Model file for the job. Use its own axes, mm. A direction names the side the tool comes from. Give positions to 0.01 mm unless a question says otherwise; leave off trailing zeros. Order: outer loops, then holes, each group sorted by start corner. A loop starts at its lowest first (then second) coordinate and runs counter-clockwise, first axis right, second up. Notation, with made-up numbers: (3.25, -21.5) -> (54.25, -21.5) arc R20 cw to (54.25, 4.5) -> close; hole circle Ø10 at (64.5, -9). An arc over 180 degrees is marked (long way). Answer in a Markdown table with one row per item. Add a question column.
from build123d import *

# Parameters (mm, degrees)
F0_W     = 20
F0_H     = 20
F0_W_2   = 10
F0_H_2   = 10
F1_DEPTH = 2.5
F2_ANGLE = 90


with BuildPart() as f1:
    # F0 (on Front) → F1 (new body)
    with BuildSketch(Plane.XZ):
        Rectangle(F0_W, F0_H)
        Rectangle(F0_W_2, F0_H_2, mode=Mode.SUBTRACT)
    extrude(amount=F1_DEPTH)


with BuildPart() as f1_1:
    # F2: moved
    add(f1.part.rotate(Axis((0, -2.5, 10), (-1, 0, 0)), F2_ANGLE))


solid = f1_1.part
Item 1: Which spindle directions (+Z, -Z, +X, -X, +Y, -Y) get a long thin tool onto all of the face, cutting with end or side? Do faces 5 (the flat face through (0, -17.5, 9)), 6 (the flat face through (0, -6, 7.5)). Say none if no direction does.
Item 2: Saw through at A-A on x = 1. List the corners of the cut face in (y, z).
Item 3: Saw through at B-B on z = 9.4. List the corners of the cut face in (x, y), plus the area to 3 significant figures.
Item 4: Wall check: line 1 (X direction, y = -8.25, z = 9.05); line 2 (Y direction, x = -2, z = 9.05). Give the ranges that are in metal, low to high.
Item 5: Saw through at C-C on y = -10.75. List the corners of the cut face in (x, z).
Item 6: Two-plate mould, pull along Y, no slides. Class faces 1 (the flat face through (0, -2.5, 9)), 2 (the flat face through (-10, -13, 9)), 3 (the flat face through (-5, -13, 9)), 4 (the flat face through (0, -7.5, 9)): pulls with the +Y half, pulls with the -Y half, needs draft (parallel to the pull), parting line crosses it, or undercut.
Evaluation:
| question | item | result |
|---|---|---|
| 1 | face 5 | +Z, -Z |
| 1 | face 6 | -Z, +X, -X, +Y, -Y |
| 2 | outline | (-22.5, 7.5) -> (-17.5, 7.5) -> (-17.5, 10) -> (-22.5, 10) -> close; (-7.5, 7.5) -> (-2.5, 7.5) -> (-2.5, 10) -> (-7.5, 10) -> close |
| 3 | outline | (-10, -22.5) -> (10, -22.5) -> (10, -2.5) -> (-10, -2.5) -> close; hole (-5, -17.5) -> (5, -17.5) -> (5, -7.5) -> (-5, -7.5) -> close |
| 3 | area | 300 mm2 |
| 4 | line 1 | x = -10 to -5, 5 to 10 |
| 4 | line 2 | y = -22.5 to -17.5, -7.5 to -2.5 |
| 5 | outline | (-10, 7.5) -> (-5, 7.5) -> (-5, 10) -> (-10, 10) -> close; (5, 7.5) -> (10, 7.5) -> (10, 10) -> (5, 10) -> close |
| 6 | face 1 | pulls with the +Y half |
| 6 | face 2 | needs draft |
| 6 | face 3 | undercut |
| 6 | face 4 | undercut |
